The listing builds one solid part. Answer for the finished solid, in the listing's coordinates (mm). Coordinates: 2 decimals unless noted, no trailing zeros. Order: outer loops, then holes, each group sorted by start corner. A loop starts at its lowest first (then second) coordinate and runs counter-clockwise, first axis right, second up. Notation, with made-up numbers: (49, 50.5) -> (84, 50.5) arc R12 cw to (84, 61.5) -> close; hole circle Ø11 at (23, 6). An arc over 180 degrees is marked (long way). One line per question, with ' | ' between items.
from build123d import *

# Parameters (mm, degrees)
SKETCH_R  = 17.5
PAD_DEPTH = 10


with BuildPart() as part:
    # Sketch → Pad (new body)
    with BuildSketch(Plane.XZ):
        Polygon((333.067415, 0), (432.926608, 99.859193), (0, 99.859193), (0, 0), align=None)
        with Locations((44.45, 49.929597)):
            Circle(SKETCH_R, mode=Mode.SUBTRACT)
    extrude(amount=PAD_DEPTH)


solid = part.part
Item 1: Section D-D, the plane x = 399.5 is taken. Give the vertices of the cut face in (y, z), plus the area to 3 significant figures.
Computed values:
outline: (-10, 66.43) -> (0, 66.43) -> (0, 99.86) -> (-10, 99.86) -> close | area: 334 mm^2
Item 2: Section C-C, the plane y = -8 is taken. Give the vertices of the cut face in (x, z), plus the area to 3 significant figures.
Computed values:
outline: (0, 0) -> (333.07, 0) -> (432.93, 99.86) -> (0, 99.86) -> close; hole circle Ø35 at (44.45, 49.93) | area: 37,300 mm^2
Item 3: Find the intervals of material crossed by L1, parallel to Z at x = 44.45, y = -4.75; L2, parallel to X at y = -2, z = 35.5; L3, parallel to X at y = -1.75, z = 50, in increasing order.
Computed values:
L1: z = 0 to 32.43, 67.43 to 99.86 | L2: x = 0 to 34.55, 54.35 to 368.57 | L3: x = 0 to 26.95, 61.95 to 383.07
Item 4: Section A-A, the plane x = 44.45 is taken. Give the vertices of the cut face in (y, z), plus the area to 3 significant figures.
Computed values:
outline: (-10, 0) -> (0, 0) -> (0, 32.43) -> (-10, 32.43) -> close; (-10, 67.43) -> (0, 67.43) -> (0, 99.86) -> (-10, 99.86) -> close | area: 649 mm^2
Item 5: Section B-B, the plane z = 63.5 is taken. Give the vertices of the cut face in (x, y).
Computed values:
outline: (0, -10) -> (33.4, -10) -> (33.4, 0) -> (0, 0) -> close; (55.5, -10) -> (396.57, -10) -> (396.57, 0) -> (55.5, 0) -> close
Item 6: Each of these flat-tipped pins is pushed along its axis until it touches: pin 1 Ø4 at (y, z) = (-3.5, 52.5) entering from +X; pin 2 Ø2 at (x, y) = (353.5, -3.5) entering from -Z; pin 3 Ø1.5 at (y, z) = (-5, 81.5) entering from +X. Where does it stop, or does it pass through?
Computed values:
pin 1: stops at x = 387.57 | pin 2: stops at z = 19.43 | pin 3: stops at x = 415.32
Item 7: Determine the mould class of faces 1 (the face through (40.656, -4.93, 32.846)), 2 (the face through (213, -10, 51)), 3 (the face through (382.3, -4.93, 49.23)), 4 (the face through (0, -5, 51)) for opening direction X: pulls with the +X half, pulls with the -X half, needs draft (parallel to the pull), parting line crosses it, or undercut.
Computed values:
face 1: undercut | face 2: needs draft | face 3: pulls with the +X half | face 4: pulls with the -X half
